```python
from build123d import *

# Parameters (mm, degrees)
EXTRUDE_1_DEPTH     = 200
SKETCH_2_R          = 1.45
CUT_EXTRUDE_1_DEPTH = 207.188353614
CUT_EXTRUDE_2_DEPTH = 207.188353614
FILLET_1_R          = 10
CHAMFER_START       = 36
CHAMFER_1_OUTLINE_W = 8
CHAMFER_1_OUTLINE_H = 200
CHAMFER_1_DEPTH     = 2.349513284
FILLET_2_R          = 6


with BuildPart() as part:
    # Эскиз1 → Бобышка-Вытянуть1 (new body)
    with BuildSketch(Plane.XY):
        with BuildLine():
            Line((25.256912811, 27.718916921), (27.395437576, 35.7))
            ThreePointArc((27.395437576, 35.7), (31.532369241, 32.10466773), (35.201522214, 28.033066792))
            Line((35.201522214, 28.033066792), (29.04384005, 23.721411323))
            ThreePointArc((29.04384005, 23.721411323), (27.223848976, 25.789766322), (25.256912811, 27.718916921))
        make_face()
    extrude(amount=EXTRUDE_1_DEPTH)

    # Эскиз2 → Вырез-Вытянуть1 (cut, through all)
    with BuildSketch(Plane.XY.offset(200)):
        with Locations((28.793836633, 31.259638065)):
            Circle(SKETCH_2_R)
    extrude(amount=-CUT_EXTRUDE_1_DEPTH, mode=Mode.SUBTRACT)

    # Эскиз4 → Вырез-Вытянуть2 (cut, through all)
    with BuildSketch(Plane.XY.offset(200)):
        with BuildLine():
            Line((29.156742817, 28.750319078), (30.957117515, 29.673853967))
            ThreePointArc((30.957117515, 29.673853967), (32.031639738, 28.118803021), (33.047614071, 26.524884074))
            Line((33.047614071, 26.524884074), (31.406028194, 25.375433268))
            ThreePointArc((31.406028194, 25.375433268), (30.316432625, 27.086234289), (29.156742817, 28.750319078))
        make_face()
    extrude(amount=-CUT_EXTRUDE_2_DEPTH, mode=Mode.SUBTRACT)

    # Скругление1
    fillet_1_edges = [part.edges().sort_by_distance(p)[0] for p in [
        (25.256912811, 27.718916921, 100),
    ]]
    fillet(fillet_1_edges, radius=FILLET_1_R)

    # Фаска1: read off the stored shape, not the designer's step
    # Фаска1 outline → Фаска1 (cut)
    with BuildSketch(Plane(origin=(0, 0, 0), x_dir=(0.7805652874719331, -0.6250742611833081, 0), z_dir=(0.6250742611833081, 0.7805652874719331, 0)).offset(CHAMFER_START)):
        with Locations((6, -100)):
            Rectangle(CHAMFER_1_OUTLINE_W, CHAMFER_1_OUTLINE_H)
    extrude(amount=CHAMFER_1_DEPTH, mode=Mode.SUBTRACT)

    # Скругление2
    fillet_2_edges = [part.edges().sort_by_distance(p)[0] for p in [
        (26.792531546, 27.67506033, 100),
    ]]
    fillet(fillet_2_edges, radius=FILLET_2_R)


solid = part.part
```
Check sheet for the modelled part. Datum: model origin and axes. Units: mm. Give positions to 0.01 mm unless a question says otherwise; leave off trailing zeros. Order: outer loops, then holes, each group sorted by start corner. A loop starts at its lowest first (then second) coordinate and runs counter-clockwise, first axis right, second up. Notation, with made-up numbers: M 60.5,59 L 110.5,59 A9 ccw 110.5,74 Z; hole C 59,-36.75 d2. An arc over 180 degrees is marked long. Answer in a Markdown table with one row per item.
1) Release check for a two-part mould opening along X. For faces 1 (the cylindrical face through (32.017, 28.141, 101.4)), 2 (the cylindrical face through (30.332, 27.063, 101.4)), 3 (the cylindrical face through (26.855, 28.551, 101.4)), 4 (the flat face through (30, 30, 0)) record: +X half, -X half, draft (parallel to the pull), parting line (faces both ways), or undercut.
Filled sheet:
| item | result |
|---|---|
| face 1 | undercut |
| face 2 | undercut |
| face 3 | -X half |
| face 4 | draft |
2) Cross-section at A-A, the plane z = 125.5. Enter the section's corners in (x, y).
Filled sheet:
| item | result |
|---|---|
| outline | M 26.4,31.38 A6 ccw 28.63,26.2 L 30.48,24.72 L 31.41,25.38 A48.84 ccw 29.16,28.75 L 30.96,29.67 A50.84 cw 33.05,26.52 L 35.2,28.03 A45 ccw 27.4,35.7 L 26.71,33.14 A10 ccw Z; hole C 28.79,31.26 d2.9 |
3) Gauge pin test, flat end, axial feed: P1, Ø1, axis at x = 34, z = 103.5, coming from the -Y side. Record the tip position at first contact, or that the pin passes through.
Filled sheet:
| item | result |
|---|---|
| P1 | stops at y = 26.84 |
4) Thickness scan on L1, parallel to Y at x = 29.75, z = 17; L2, parallel to Y at x = 29.5, z = 90; L3, parallel to Y at x = 30.75, z = 174. Record the ranges inside material, lowest first. Write a range as [from, to].
Filled sheet:
| item | result |
|---|---|
| L1 | y = [25.31, 27.92], [29.05, 30.17], [32.35, 33.76] |
| L2 | y = [25.51, 28.27], [28.93, 29.99], [32.53, 33.98] |
| L3 | y = [24.92, 26.42], [29.57, 32.85] |
